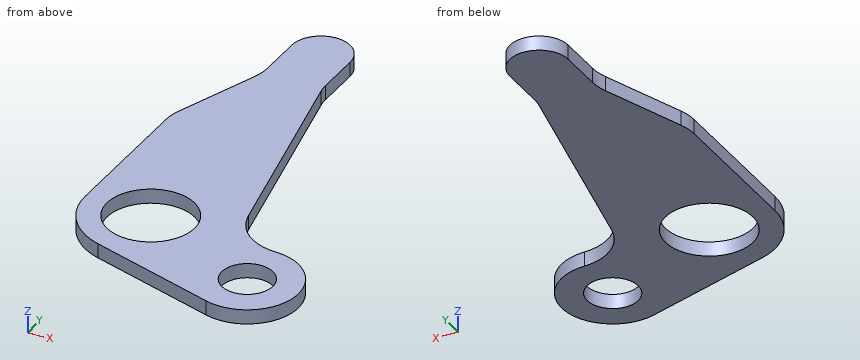
Autodesk Inventor part; units mm, degrees
ref_plane "YZ Plane" through (0, 0, 0) normal (1, 0, 0) x (0, 1, 0)
ref_plane "XZ Plane" through (0, 0, 0) normal (0, 1, 0) x (-1, 0, 0)
ref_plane "XY Plane" through (0, 0, 0) normal (0, 0, 1) x (1, 0, 0)
sketch "Sketch1" plane through (0, 0, 0) normal (0, 0, 1) x (1, 0, 0)
  line L0 (-115.9793, -35.2742) -> (-115.9793, 64.2246)
  arc A0 (-113.8324, 76.2941) -> (-115.9793, 64.2246) centre (-80.9793, 64.2246) ccw
  line L1 (-113.8324, 76.2941) -> (-93.1262, 132.6563)
  arc A1 (-93.1262, 132.6563) -> (-90.9793, 144.7258) centre (-125.9793, 144.7258) ccw
  line L2 (-90.9793, 144.7258) -> (-90.9793, 174.7258)
  arc A2 (-50.9793, 174.7258) -> (-90.9793, 174.7258) centre (-70.9793, 174.7258) ccw
  line L3 (-50.9793, 174.7258) -> (-50.9793, 144.7258)
  arc A3 (-50.9793, 144.7258) -> (-50.222, 137.4844) centre (-15.9793, 144.7258) ccw
  line L4 (-50.222, 137.4844) -> (-19.622, -7.2156)
  arc A4 (-115.9793, -35.2742) -> (-83.2704, -78.5631) centre (-70.9793, -35.2742) ccw
  line L5 (-83.2704, -78.5631) -> (5.0609, -103.6433)
  arc A5 (5.0609, -103.6433) -> (14.6207, -34.9742) centre (14.6207, -69.9742) ccw
  arc A6 (-19.622, -7.2156) -> (14.6207, -34.9742) centre (14.6207, 0.0258) ccw
  circle A7 centre (-70.9793, -35.2742) radius 30
  circle A8 centre (14.6207, -69.9742) radius 17.5
  dimension "d0" = 20
  dimension "d1" = 210
  dimension "d4" = 85.6
  dimension "d5" = 34.7
  dimension "d7" = 35
  dimension "d8" = 35
  dimension "d9" = 35
  dimension "d10" = 35
  dimension "d11" = 45
  dimension "d12" = 35
  dimension "d13" = 100
  dimension "d15" = 35
  dimension "d16" = 60
  dimension "d17" = 180
  dimension "d18" = 180
extrude "Extrusion1" add sketch "Sketch1" along normal blind 10
equation "\"d8\" = d7"
equation "\"d9\" = d7"
equation "\"d10\" = d9"
properties part number "3136 1133 81" material "Steel, Mild"
CAD build for the part. Positions are in the model's coordinates, mm. Round coordinates to 2 decimals unless told otherwise and drop trailing zeros. Write each loop counter-clockwise with the first axis right and the second up, starting at its lowest first coordinate (ties: lowest second). Pieces come first, ordered by that corner, then holes.
Item 1: Drill centre lines: L1, parallel to Y at x = 7, z = 8; L2, parallel to Y at x = -80, z = 1; L3, parallel to X at y = 123.5, z = 1.5. Where is each one in solid material? Low to high.
Filled in:
L1: y = -104.13 to -85.73, -54.22 to -34.13
L2: y = -79.49 to -63.89, -6.66 to 192.58
L3: x = -96.49 to -47.26
Item 2: Band-saw the part on D-D on y = 166.5. Write the cut outline in (x, z).
Filled in:
outline: (-90.98, 0) - (-50.98, 0) - (-50.98, 10) - (-90.98, 10) - close
Item 3: Band-saw the part on C-C on z = 3.5. Write the cut outline in (x, y), then the cut area to 4 significant figures.
Filled in:
outline: (-115.98, -35.27) arc R45 ccw to (-83.27, -78.56) - (5.06, -103.64) arc R35 ccw (long way) to (14.62, -34.97) arc R35 cw to (-19.62, -7.22) - (-50.22, 137.48) arc R35 cw to (-50.98, 144.73) - (-50.98, 174.73) arc R20 ccw to (-90.98, 174.73) - (-90.98, 144.73) arc R35 cw to (-93.13, 132.66) - (-113.83, 76.29) arc R35 ccw to (-115.98, 64.22) - close; hole circle Ø60 at (-70.98, -35.27); hole circle Ø35 at (14.62, -69.97)
area: 20,750 mm2
Item 4: Band-saw the part on B-B on x = 1.5. Write the cut outline in (y, z), then the cut area to 3 significant figures.
Filled in:
outline: (-102.63, 0) - (-81.55, 0) - (-81.55, 10) - (-102.63, 10) - close; (-58.39, 0) - (-32.42, 0) - (-32.42, 10) - (-58.39, 10) - close
area: 471 mm2
Item 5: Drop flat-ended pins along their axis: pin 1 Ø1 at (x, z) = (-58.5, 8) entering from +Y; pin 2 Ø3 at (x, z) = (-1, 2.5) entering from -Y; pin 3 Ø1 at (x, z) = (20, 2.5) entering from +Y. Give the stop position or say it passes through.
Filled in:
pin 1: stops at y = 190.74
pin 2: stops at y = -102.35
pin 3: stops at y = -35.32
Item 6: Band-saw the part on A-A on y = -20.5. Write the cut outline in (x, z), then the cut area to 3 significant figures.
Filled in:
outline: (-115.98, 0) - (-97.09, 0) - (-97.09, 10) - (-115.98, 10) - close; (-44.87, 0) - (-13.73, 0) - (-13.73, 10) - (-44.87, 10) - close
area: 500 mm2
